Autodesk Inventor part; units mm, degrees
ref_plane "WeldJoint" through (0, 0, -10) normal (0.5299, -0.848, 0) x (0, 0, 1)
ref_plane "Outer" through (0, 0, -10) normal (0.454, -0.891, 0) x (0, 0, 1)
ref_plane "Clock_Feeder" through (0, 0, -10) normal (0.7071, 0.7071, 0) x (0, 0, 1)
sketch "Sketch13" plane through (0, 0, 0) normal (0, 0, 1) x (1, 0, 0)
  circle A0 centre (0, 0) radius 425 construction
  line L0 (0, 0) -> (0, -425)
  line L1 (0, 0) -> (-360.4204, -225.2157)
  line L2 (0, 0) -> (300.5204, -300.5204)
  line L3 (0, 0) -> (0, -425)
  line L4 (0, 0) -> (0, -425)
  line L5 (0, 0) -> (-378.6778, -192.946)
  arc A1 (-360.4204, -225.2157) -> (0, -425) centre (0, 0) ccw
  dimension "d53" = 850
  dimension "d54" = 58
  dimension "d55" = 0
  dimension "d56" = 0
  dimension "d57" = 315
  dimension "d58" = 63
ref_plane "WeldJoint" through (0, 0, -10) normal (0.5299, -0.848, 0) x (0, 0, 1)
ref_plane "Outer" through (0, 0, -10) normal (0.454, -0.891, 0) x (0, 0, 1)
ref_plane "Clock_Feeder" through (0, 0, -10) normal (0.7071, 0.7071, 0) x (0, 0, 1)
ref_plane "Charging" through (0, 0, -10) normal (1, 0, 0) x (0, 0, 1)
ref_plane "Accsess" through (0, 0, -10) normal (1, 0, 0) x (0, 0, 1)
sketch "Sketch14" plane through (0, 0, -10) normal (0.5299, -0.848, 0) x (0, 0, 1)
  line L0 (1410, 419) -> (10, 419)
  line L1 (10, 419) -> (10, 425)
  line L2 (10, 425) -> (1410, 425)
  line L3 (1410, 425) -> (1410, 419)
  line L4 (10, 0) -> (825.0673, 0)
  point P0 (10, 422)
  dimension "d59" = 1400
  dimension "d60" = 6
  dimension "d61" = 850
revolve "Revolution2" add sketch "Sketch14" angle 359.9 about axis through (0, 0, 0) along (0, 0, 1)
sketch "Sketch AnglePlane_Feeder" plane through (0, 0, -10) normal (0.7071, 0.7071, 0) x (0, 0, 1)
  line L0 (10, -425) -> (10, 425)
  line L1 (10, 0) -> (1210, 0)
  line L2 (1210, 0) -> (1210, 425)
  line L3 (1210, 425) -> (10, 425)
  line L4 (10, 425) -> (10, 0)
  point P0 (10, -95.6042)
  point P1 (10, -96.3268)
  dimension "d63" = 850
  dimension "d64" = 90
  dimension "frd_hght" = 1200
ref_plane "AnglePlane_Feeder" through (0, 0, 1200) normal (0.7071, -0.7071, 0) x (0.7071, 0.7071, 0)
sketch "Sketch16" plane through (0, 0, 1200) normal (0.7071, -0.7071, 0) x (0.7071, 0.7071, 0)
  circle A0 centre (0, 0) radius 29.5
  point P0 (0, -1200)
  point P1 (0, 0)
  point P2 (0, 0)
  point P3 (0, 0)
  dimension "d66" = 59
extrude "Extrusion7" cut sketch "Sketch16" along normal through all
ref_plane "Work Plane16" through (0, 0, 0) normal (0, -1, 0) x (1, 0, 0)
sketch "Sketch17" plane through (0, 0, 0) normal (0, -1, 0) x (1, 0, 0)
  circle A0 centre (0, 408.5) radius 268.5
  line L0 (0, 140) -> (-495.5727, 140)
  point P0 (0, 0)
  dimension "d69" = 537
  dimension "d71" = 140
extrude "Extrusion8" cut sketch "Sketch17" along normal through all
sketch "Sketch19" plane through (0, 0, -10) normal (1, 0, 0) x (0, 0, 1)
  line L0 (10, 0) -> (1110, 0)
  line L1 (1110, 0) -> (1110, 425)
  line L2 (1110, 425) -> (10, 425)
  line L3 (10, 425) -> (10, 0)
  dimension "d74" = 1100
  dimension "d76" = 850
  dimension "d77" = 90
ref_plane "Work Plane18" through (0, 0, 1100) normal (0, -1, 0) x (1, 0, 0)
sketch "Sketch20" plane through (0, 0, 1100) normal (0, -1, 0) x (1, 0, 0)
  line L0 (-103.5, 0) -> (103.5, 0)
  line L1 (103.5, 0) -> (103.5, 125)
  line L2 (103.5, 125) -> (-103.5, 125)
  line L3 (-103.5, 125) -> (-103.5, 0)
  point P0 (0, -1100)
  point P1 (0, 0)
  point P2 (0, 0)
  point P3 (0, 0)
  point P4 (0, 0)
  dimension "d78" = 207
  dimension "d79" = 125
extrude "Extrusion9" cut sketch "Sketch20" along normal through all
equation "\"BendRadius\" = Thickness"
equation "\"BendReliefWidth\" = Thickness"
equation "\"BendReliefDepth\" = 0.5 * Thickness"
equation "\"CornerReliefSize\" = 4 * Thickness"
equation "\"MinimumRemnant\" = 2 * Thickness"
equation "\"TransitionRadius\" = BendRadius"
equation "\"JacobiRadiusSize\" = BendRadius"
equation "\"GapSize\" = Thickness"
equation "\"Feeder_horisont_angle\" = 0"
equation "\"Hatch_Accsess_diameter\" = 535"
equation "\"Clock_Accsess_angle\" = 0"
equation "\"Clock_Charging_agnle\" = 0"
equation "\"Clock_Feeder_angle\" = 315deg"
equation "\"Clock_Outer_angle\" = 63deg"
equation "\"Clock_WeldJoint_angle\" = 58deg"
properties part number "PNS 9110 main Shell D 940" material "Steel"
Model file for the job. Use its own axes, mm. A direction names the side the tool comes from. Coordinates: 2 decimals unless noted, no trailing zeros. Loops run counter-clockwise (first coordinate to the right, second up) from the corner with the lowest first, then second, coordinate; pieces in that order, holes last. Notation, with made-up numbers: (19.25, 55.25) -> (36.25, 55.25) arc R32 ccw to (36.25, 81.25) -> close; hole circle Ø6 at (1, -37). An arc over 180 degrees is marked (long way). Use one line per item in the form item = value. Start each with the question number.
(1) Cut at D-D on y = -372. Give the cut face in (x, z).
(2) Flat gauge pins, fed straight in: pin 1 (12 mm diameter, centred on y = 82.5, z = 311, fed in from +X); pin 2 (4 mm diameter, centred on x = -112, z = 310, fed in from -Y); pin 3 (15 mm diameter, centred on x = -23, y = -411.5, fed in from -Z); pin 4 (5 mm diameter, centred on y = 282.5, z = 929.5, fed in from -X). Where does each tip first touch, or does it go through?
(3) Pull direction Y, two halves, no side cores. Call faces 1 (the flat face through (-404, 116, 1400)), 2 (the cylindrical face through (149.397, 397.876, 709.8)), 3 (the cylindrical face through (112.27, 403.68, 690.2)), 4 (the cylindrical face through (317.27, -278.73, 1211.3)): pulls with the +Y half, pulls with the -Y half, needs draft (parallel to the pull), parting line crosses it, or undercut.
(4) Cut at B-B on y = 0. Give the cut face in (x, z), and give its area (3 significant figures).
(5) Cut at C-C on x = 0. Give the cut face in (y, z).
(6) Probe probe 1 along Y at (x, z) = (0, 971); probe 2 along Y at (x, z) = (0, 564). List the from-to ranges inside material, lowest first. Write a range as from..to.
(7) Tool access for faces 5 (the cylindrical face through (187.099, -376.915, 215.922)), 6 (the flat face through (-404, 116, 0)): list every direction of +Z, -Z, +X, -X, +Y, -Y with a clear straight run to the whole face (end or side of a thin tool).
(8) Cut at A-A on z = 1135. Give the cut face in (x, y).
Values:
q1.outline = (-205.53, 0) -> (-192.81, 0) -> (-192.81, 221.64) arc R268.5 cw to (-205.53, 235.72) -> close; (-205.53, 581.28) arc R268.5 cw to (-192.81, 595.36) -> (-192.81, 1400) -> (-205.53, 1400) -> close; (192.81, 0) -> (205.53, 0) -> (205.53, 235.72) arc R268.5 cw to (192.81, 221.64) -> close; (192.81, 595.36) arc R268.5 cw to (205.53, 581.28) -> (205.53, 1400) -> (192.81, 1400) -> close
q2.pin_1 = 418.06
q2.pin_2 = 403.19
q2.pin_3 = 0
q2.pin_4 = -319.73
q3.face_1 = needs draft
q3.face_2 = parting line crosses it
q3.face_3 = undercut
q3.face_4 = undercut
q4.outline = (-425, 0) -> (-419, 0) -> (-419, 1400) -> (-425, 1400) -> close; (419, 0) -> (425, 0) -> (425, 1400) -> (419, 1400) -> close
q4.area = 16,800 mm2
q5.outline = (-425, 0) -> (-419, 0) -> (-419, 140) -> (-425, 140) -> close; (-425, 677) -> (-419, 677) -> (-419, 1100) -> (-425, 1100) -> close; (-425, 1225) -> (-419, 1225) -> (-419, 1400) -> (-425, 1400) -> close; (419, 0) -> (425, 0) -> (425, 1400) -> (419, 1400) -> close
q6.probe_1 = -425..-419, 419..425
q6.probe_2 = 419..425
q7.face_5 = -Y
q7.face_6 = -Z, +X, -X, +Y, -Y
q8.outline = (-360.81, -224.59) -> (-355.72, -221.42) arc R419 cw (long way) to (103.5, -406.02) -> (103.5, -412.2) arc R425 ccw (long way) to start; (-360.42, -225.22) arc R425 ccw to (-103.5, -412.2) -> (-103.5, -406.02) arc R419 cw to (-355.33, -222.04) -> close
